For this review, use the dimensioned drawing (mm, ordinates from the lowest corner) and the shaded views. Coordinates: 2 decimals unless noted, no trailing zeros. Loops run counter-clockwise (first coordinate to the right, second up) from the corner with the lowest first, then second, coordinate; pieces in that order, holes last. Notation, with made-up numbers: (64.5, 42) -> (103.5, 42) arc R20 ccw to (103.5, 80) -> close; hole circle Ø4 at (23.5, 87.25). An arc over 180 degrees is marked (long way). Use one line per item in the form item = value. Start each with the question number.
1. Consider section C-C (y = 57). State the section outline as (x, z) points, then the cut area to 3 significant figures.
2. Wall thickness on line 1 (Z direction, x = 4.55, y = 92); line 2 (Y direction, x = 2.7, z = 167); line 3 (Z direction, x = 1.1, y = 72): over which ranges is each line inside the solid? List them lowest first. Write a range as from..to.
3. Consider section D-D (x = 3.7). State how many separate pieces and enclosed holes the cut face has, then the cut area to 3 significant figures.
4. For pin 1 (1.8 mm diameter, centred on x = 3.5, y = 52.5, fed in from -Z), flat-tipped, find the tip position at first contact; note if it passes through.
5. Consider section B-B (z = 41). State the section outline as (x, y) points.
6. Consider section A-A (y = 43). State the section outline as (x, z) points, then the cut area to 3 significant figures.
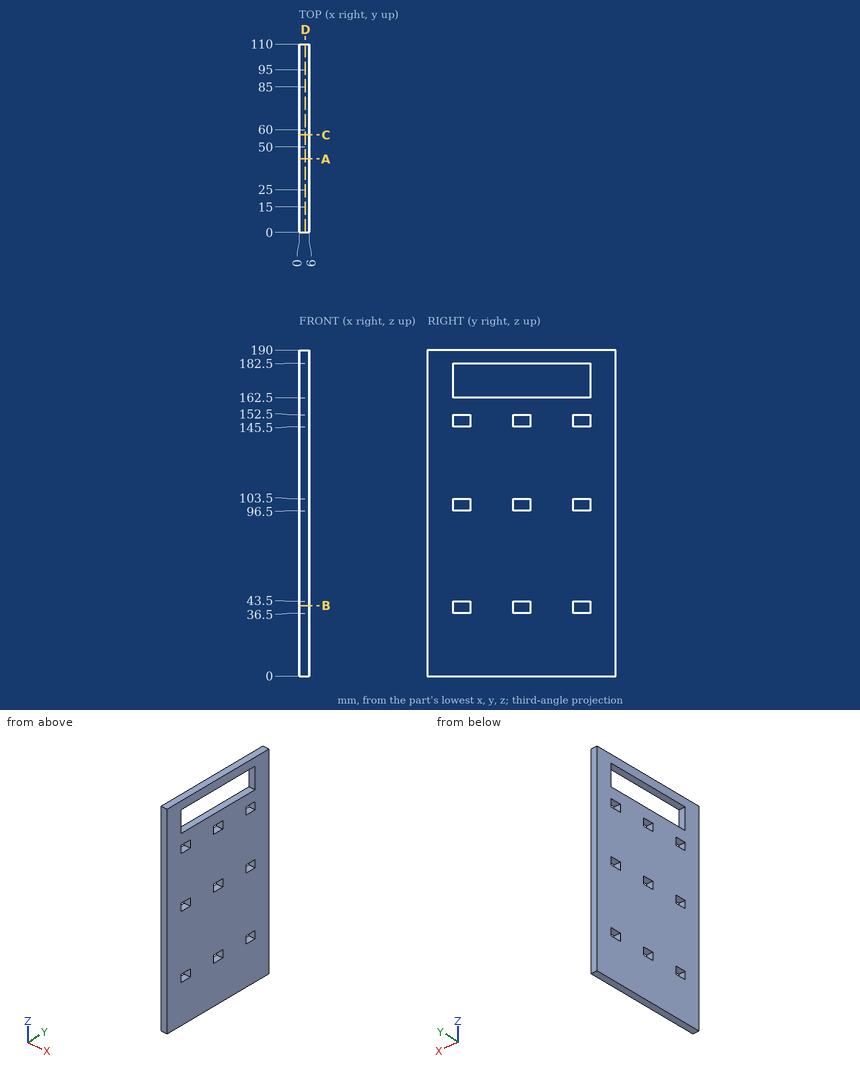
Geometry check:
q1.outline = (0, 0) -> (6, 0) -> (6, 36.5) -> (0, 36.5) -> close; (0, 43.5) -> (6, 43.5) -> (6, 96.5) -> (0, 96.5) -> close; (0, 103.5) -> (6, 103.5) -> (6, 145.5) -> (0, 145.5) -> close; (0, 152.5) -> (6, 152.5) -> (6, 162.5) -> (0, 162.5) -> close; (0, 182.5) -> (6, 182.5) -> (6, 190) -> (0, 190) -> close
q1.area = 894 mm²
q2.line_1 = 0..36.5, 43.5..96.5, 103.5..145.5, 152.5..162.5, 182.5..190
q2.line_2 = 0..15, 95..110
q2.line_3 = 0..162.5, 182.5..190
q3.separate_pieces = 1
q3.enclosed_holes = 10
q3.area = 18,700 mm²
q4.pin_1 = 0
q5.outline = (0, 0) -> (6, 0) -> (6, 15) -> (0, 15) -> close; (0, 25) -> (6, 25) -> (6, 50) -> (0, 50) -> close; (0, 60) -> (6, 60) -> (6, 85) -> (0, 85) -> close; (0, 95) -> (6, 95) -> (6, 110) -> (0, 110) -> close
q6.outline = (0, 0) -> (6, 0) -> (6, 162.5) -> (0, 162.5) -> close; (0, 182.5) -> (6, 182.5) -> (6, 190) -> (0, 190) -> close
q6.area = 1,020 mm²
